```python
from build123d import *

# Parameters (mm, degrees)
SKETCH1_W                     = 7
SKETCH1_H                     = 40
F_8_0_8_DIAMETER_HOLE1_D      = 8
F_4_0_4_DIAMETER_HOLE1_REACH  = 37.623
F_4_0_4_DIAMETER_HOLE1_BORE_R = 2


with BuildPart() as part:
    # Sketch1 → Revolve1 (revolve)
    with BuildSketch(Plane.XZ, mode=Mode.PRIVATE) as revolve1_sk:
        with Locations((3.5, 20)):
            Rectangle(SKETCH1_W, SKETCH1_H)
    revolve(revolve1_sk.sketch.rotate(Axis((0, 0, 40), (0, 0, -1)), 180), axis=Axis((0, 0, 40), (0, 0, -1)))

    # Ø8.0 (8) Diameter Hole1 (through all)
    with Locations(Plane.XY.offset(40)):
        with Locations((0, 0)):
            Hole(F_8_0_8_DIAMETER_HOLE1_D / 2)

    # Ø4.0 (4) Diameter Hole1 bore (on position points) → Ø4.0 (4) Diameter Hole1 (cut, up to next)
    with BuildSketch(Plane(origin=(0, 7, 32), x_dir=(1, 0, 0), z_dir=(0, 1, 0)), mode=Mode.PRIVATE) as f_4_0_4_diameter_hole1_sk1:
        Circle(F_4_0_4_DIAMETER_HOLE1_BORE_R)
    f_4_0_4_diameter_hole1_tool1 = extrude(f_4_0_4_diameter_hole1_sk1.sketch, amount=-F_4_0_4_DIAMETER_HOLE1_REACH, mode=Mode.PRIVATE) & part.part
    add(f_4_0_4_diameter_hole1_tool1.solids().sort_by_distance((0, 7, 32))[0], mode=Mode.SUBTRACT)


solid = part.part
```
Input: part model. Units: mm. Frame: model coordinates. A direction names the side the tool comes from. Coordinates: 2 decimals unless noted, no trailing zeros. Loops run counter-clockwise (first coordinate to the right, second up) from the corner with the lowest first, then second, coordinate; pieces in that order, holes last. Notation, with made-up numbers: M 68,18 L 102,18 A26 ccw 102,46 Z; hole C 32.25,68 d4. An arc over 180 degrees is marked long. One line per item, written item: value.
(1) Reachability of faces 1 (the flat face through (3, -3, 40)), 2 (the cylindrical face through (0.923, 5.257, 33.774)) from +Z, -Z, +X, -X, +Y, -Y: full face, straight path, thin tool, end or side. Return the list, or none.
Filled in:
face 1: +Z, +X, -X, +Y, -Y
face 2: +Y
(2) Section D-D (y = -3.25). Output: boundary loops of the cut face in (x, z), and give its area (3 significant figures).
Filled in:
outline: M -6.2,0 L -2.33,0 L -2.33,40 L -6.2,40 Z; M 2.33,0 L 6.2,0 L 6.2,40 L 2.33,40 Z
area: 309 mm^2
(3) Section C-C (z = 25.5). Output: boundary loops of the cut face in (x, y).
Filled in:
outline: C 0,0 d14; hole C 0,0 d8
(4) Section B-B (x = 0). Output: boundary loops of the cut face in (y, z).
Filled in:
outline: M -7,0 L -4,0 L -4,40 L -7,40 Z; M 4,0 L 7,0 L 7,30 L 4,30 Z; M 4,34 L 7,34 L 7,40 L 4,40 Z
(5) Section A-A (y = 0). Output: boundary loops of the cut face in (x, z).
Filled in:
outline: M -7,0 L -4,0 L -4,40 L -7,40 Z; M 4,0 L 7,0 L 7,40 L 4,40 Z
(6) Pull-direction query (X, two-part tool) for faces 3 (the flat face through (3, -3, 0)), 4 (the cylindrical face through (-3.23, -6.21, 20.28)), 5 (the cylindrical face through (0.867, -3.905, 19.72)); classes: +X half, -X half, draft (parallel to the pull), parting line (faces both ways), or undercut.
Filled in:
face 3: draft
face 4: parting line
face 5: undercut
(7) Pin query (flat end, axial travel): pin 1 (2 mm diameter, centred on x = 3, z = 30.5, fed in from -Y); pin 2 (3 mm diameter, centred on x = -5.5, y = -3, fed in from -Z); pin 3 (1 mm diameter, centred on y = 5, z = 16.5, fed in from -X); pin 4 (2 mm diameter, centred on y = 1.5, z = 8, fed in from +X). Return the tip coordinate at first contact, or that it passes through.
Filled in:
pin 1: y = -6.71
pin 2: z = 0
pin 3: x = -5.36
pin 4: x = 6.98
(8) Line query: line 1 along Y through (x, z) = (-0.25, 8); line 2 along Z through (x, y) = (0, 5.75); line 3 along Y through (x, z) = (-2, 7). Output: solid intervals per line, ascending. Write a range as from..to.
Filled in:
line 1: -7..-3.99, 3.99..7
line 2: 0..30, 34..40
line 3: -6.71..-3.46, 3.46..6.71
